Here's how the part is built. I have some questions about the finished solid (model axes, mm). Give positions to 0.01 mm unless a question says otherwise; leave off trailing zeros. Write each loop counter-clockwise with the first axis right and the second up, starting at its lowest first coordinate (ties: lowest second). Pieces come first, ordered by that corner, then holes. Notation, with made-up numbers: (86, 58) - (118, 58) arc R31 cw to (118, 93) - close; hole circle Ø2 at (-40, 7). An arc over 180 degrees is marked (long way). Write each question's results on one line, items separated by ' | '. Start each with the question number.
Item 1: Will these pins go through, and if not, where does the flat tip stop? P1, Ø1, axis at y = 179.5, z = -1, coming from the -X side; P2, Ø1.5, axis at x = 1.5, z = 1, coming from the +Y side; P3, Ø1, axis at x = 8, y = 173, coming from the +Z side; P4, Ø7, axis at x = 16.55, y = 81.5, coming from the -Z side.
Item 2: Please list where these lines run through material, in increasing order: line 1 along Y through (x, z) = (20, -0.75); line 2 along X through (y, z) = (152, -0.2); line 3 along Y through (x, z) = (-8, 0.4).
Item 3: Suppose I cut it at A-A on z = 0.15. List the corners of the cut face in (x, y) for me, then the cut area to 3 significant figures.
Item 4: We'd pull the mould along Y, two halves only. Please class faces 1 (the cylindrical face through (-8.095, 217.928, 0.01)), 2 (the cylindrical face through (20.37, 91.6, -0.01)), 3 (the cylindrical face through (-4.86, 232.49, -0.02)): +Y half, -Y half, draft (parallel to the pull), parting line (faces both ways), or undercut.
```python
from build123d import *

# Parameters (mm, degrees)
SKETCH2_R           = 4.5
BOSS_EXTRUDE1_DEPTH = 1.5
FILLET2_R           = 15
FILLET1_R           = 0.8


with BuildPart() as part:
    # Sketch2 → Boss-Extrude1 (new, symmetric)
    with BuildSketch(Plane.XY):
        with BuildLine():
            Line((1.274716536, 220.943357999), (19.912187432, 89.850027402))
            ThreePointArc((19.912187432, 89.850027402), (17.820843773, 72.589598754), (11.001786186, 88.583240273))
            Line((11.001786186, 88.583240273), (-7.635684711, 219.67657087))
            ThreePointArc((-7.635684711, 219.67657087), (-5.544341051, 236.936999518), (1.274716536, 220.943357999))
        make_face()
        with Locations((-4.277553922, 228.026598272)):
            Circle(SKETCH2_R, mode=Mode.SUBTRACT)
        with Locations((16.554056644, 81.5)):
            Circle(SKETCH2_R, mode=Mode.SUBTRACT)
    extrude(amount=BOSS_EXTRUDE1_DEPTH, both=True)

    # Fillet2
    fillet2_edges = [part.edges().sort_by_distance(p)[0] for p in [
        (-7.635684711, 219.67657087, 0),
        (1.274716536, 220.943357999, 0),
        (19.912187432, 89.850027402, 0),
        (11.001786186, 88.583240273, 0),
    ]]
    fillet(fillet2_edges, radius=FILLET2_R)

    # Fillet1
    fillet1_edges = [part.edges().sort_by_distance(p)[0] for p in [
        (-5.544341051, 236.936999518, -1.5),
        (-5.544341051, 236.936999518, 1.5),
        (10.593451984, 155.396692701, -1.5),
        (10.593451984, 155.396692701, 1.5),
        (17.820843773, 72.589598754, -1.5),
        (17.820843773, 72.589598754, 1.5),
        (1.683050738, 154.129905572, -1.5),
        (1.683050738, 154.129905572, 1.5),
        (2.213746014, 219.456683126, -1.5),
        (2.213746014, 219.456683126, 1.5),
        (20.399664536, 91.539507977, -1.5),
        (20.399664536, 91.539507977, 1.5),
        (10.062756708, 90.069915146, -1.5),
        (10.062756708, 90.069915146, 1.5),
        (-8.123161814, 217.987090295, -1.5),
        (-8.123161814, 217.987090295, 1.5),
    ]]
    fillet(fillet1_edges, radius=FILLET1_R)


solid = part.part
```
Checked values:
1) P1: stops at x = -1.98 | P2: stops at y = 235.47 | P3: stops at z = 1.47 | P4: passes through
2) line 1: y = 73.19 to 78.61, 84.39 to 92.43 | line 2: x = 1.99 to 11.08 | line 3: y = 217.73 to 225.5, 230.56 to 236.22
3) outline: (-10.78, 221.8) arc R15 cw to (-6.76, 213.54) - (10.13, 94.72) arc R15 cw to (8.58, 85.67) arc R9 ccw (long way) to (23.06, 87.72) arc R15 cw to (19.04, 95.99) - (2.15, 214.81) arc R15 cw to (3.7, 223.86) arc R9 ccw (long way) to start; hole circle Ø9 at (-4.28, 228.03); hole circle Ø9 at (16.55, 81.5) | area: 1,570 mm^2
4) face 1: -Y half | face 2: +Y half | face 3: undercut
